```python
from build123d import *

# Parameters (mm, degrees)
F0_W      = 914.4
F0_H      = 812.8
F0_W_2    = 762
F0_H_2    = 609.6
F1_DEPTH  = 63.5
F2_W      = 914.4
F2_H      = 812.8
F2_W_2    = 762
F2_H_2    = 660.4
F3_DEPTH  = 1219.2
F5_DEPTH  = 812.8
F5_FACE_W = 762
F5_FACE_H = 76.2
F7_W      = 762
F7_H      = 282.4884019335
F9_DEPTH  = 76.2
F10_W     = 63.5
F10_H     = 76.2
F12_W     = 762
F12_H     = 279.4
F13_DEPTH = 88.9
F14_START = -330.2
F14_DEPTH = 152.4
F15_R     = 101.6
F16_DEPTH = 76.2
F17_DEPTH = 76.2


with BuildPart() as f1:
    # F0 (on Top) → F1 (new body)
    with BuildSketch(Plane.XY):
        Rectangle(F0_W, F0_H)
        Rectangle(F0_W_2, F0_H_2, mode=Mode.SUBTRACT)
        Rectangle(F0_W_2, F0_H_2)
    extrude(amount=F1_DEPTH)

    # F2 (on face) → F3 (join)
    with BuildSketch(Plane.XY.offset(63.5)):
        Rectangle(F2_W, F2_H)
        Rectangle(F2_W_2, F2_H_2, mode=Mode.SUBTRACT)
    extrude(amount=F3_DEPTH)

    # F4 (on face) → F5 (join, through all)
    with BuildSketch(Plane.XZ.offset(406.4)):
        with BuildLine():
            Line((381, 1282.7), (457.2, 1282.7))
            ThreePointArc((457.2, 1282.7), (364.8558540126, 1558.2214071405), (125.1263088683, 1722.4445245014))
            Line((125.1263088683, 1722.4445245014), (63.5, 1658.3710662268))
            ThreePointArc((63.5, 1658.3710662268), (290.9935566297, 1528.6344424842), (381, 1282.7))
        make_face()
        with BuildLine():
            ThreePointArc((-125.1263088683, 1722.4445245014), (-364.8558540126, 1558.2214071405), (-457.2, 1282.7))
            Line((-457.2, 1282.7), (-381, 1282.7))
            ThreePointArc((-381, 1282.7), (-290.9935566297, 1528.6344424842), (-63.5, 1658.3710662268))
            Line((-63.5, 1658.3710662268), (-125.1263088683, 1722.4445245014))
        make_face()
        with BuildLine():
            Line((63.5, 1658.3710662268), (125.1263088683, 1722.4445245014))
            ThreePointArc((125.1263088683, 1722.4445245014), (0, 1739.9), (-125.1263088683, 1722.4445245014))
            Line((-125.1263088683, 1722.4445245014), (-63.5, 1658.3710662268))
            ThreePointArc((-63.5, 1658.3710662268), (0, 1663.7), (63.5, 1658.3710662268))
        make_face()
    extrude(amount=-F5_DEPTH)

    # F5_face (on face) → F6 (join, up to the next surface of F1)
    with BuildSketch(Plane(origin=(0, 368.3, 1282.7), x_dir=(1, 0, 0), z_dir=(0, 0, 1))):
        Rectangle(F5_FACE_W, F5_FACE_H)
    extrude(until=Until.NEXT)

    # F5_face (on face) → F8 (join, up to the next surface of F1)
    with BuildSketch(Plane(origin=(0, 368.3, 1282.7), x_dir=(1, 0, 0), z_dir=(0, 0, 1))):
        with Locations((0, -736.6)):
            Rectangle(F5_FACE_W, F5_FACE_H)
    extrude(until=Until.NEXT)

    # F7 (on face) → F9 (cut, through all)
    with BuildSketch(Plane.XZ.offset(406.4)):
        with BuildLine():
            Line((381, 1282.7), (-381, 1282.7))
            Line((-381, 1282.7), (-381, 726.9884019335))
            ThreePointArc((-381, 726.9884019335), (0, 850.9), (381, 726.9884019335))
            Line((381, 726.9884019335), (381, 1282.7))
        make_face()
        with BuildLine():
            ThreePointArc((381, 650.7884019335), (0, 774.7), (-381, 650.7884019335))
            Line((-381, 650.7884019335), (381, 650.7884019335))
        make_face()
        with Locations((0, 509.5442009667)):
            Rectangle(F7_W, F7_H)
    extrude(amount=-F9_DEPTH, mode=Mode.SUBTRACT)

    # F11: sweep along a path in F7
    with BuildLine(Plane.XZ.offset(406.4)) as f11_path:
        ThreePointArc((381, 650.7884019335), (0, 774.7), (-381, 650.7884019335))
    # F10 (on face) → F11 (sweep)
    with BuildSketch(Plane.YZ.offset(-381)):
        with Locations((-152.4, 688.8884019335)):
            Rectangle(F10_W, F10_H)
        with Locations((88.9, 688.8884019335)):
            Rectangle(F10_W, F10_H)
        with Locations((298.45, 688.8884019335)):
            Rectangle(F10_W, F10_H)
    sweep(path=f11_path.line)

    # F12 (on face) → F13 (cut)
    with BuildSketch(Plane(origin=(0, 406.4, 0), x_dir=(-1, 0, 0), z_dir=(0, 1, 0))):
        with Locations((0, 203.2)):
            Rectangle(F12_W, F12_H)
    extrude(amount=-F13_DEPTH, mode=Mode.SUBTRACT)

    # F4 (on face) → F14 (cut)
    with BuildSketch(Plane.XZ.offset(406.4).offset(F14_START)):
        with BuildLine():
            Line((63.5, 1658.3710662268), (125.1263088683, 1722.4445245014))
            ThreePointArc((125.1263088683, 1722.4445245014), (0, 1739.9), (-125.1263088683, 1722.4445245014))
            Line((-125.1263088683, 1722.4445245014), (-63.5, 1658.3710662268))
            ThreePointArc((-63.5, 1658.3710662268), (0, 1663.7), (63.5, 1658.3710662268))
        make_face()
    extrude(amount=-F14_DEPTH, mode=Mode.SUBTRACT)

    # F15 (on face) → F16 (cut, through all)
    with BuildSketch(Plane(origin=(-457.2, 0, 0), x_dir=(0, -1, 0), z_dir=(-1, 0, 0))):
        with Locations((0, 509.5442009667)):
            Circle(F15_R)
    extrude(amount=-F16_DEPTH, mode=Mode.SUBTRACT)

    # F7 (on face) → F17 (join, through all)
    with BuildSketch(Plane.XZ.offset(406.4)):
        with BuildLine():
            ThreePointArc((381, 650.7884019335), (0, 774.7), (-381, 650.7884019335))
            Line((-381, 650.7884019335), (381, 650.7884019335))
        make_face()
    extrude(amount=-F17_DEPTH)


solid = f1.part
```
The model under review builds one solid part; all positions refer to its coordinate system, in mm. A direction names the side the tool comes from. Round coordinates to 2 decimals unless told otherwise and drop trailing zeros. Loops run counter-clockwise (first coordinate to the right, second up) from the corner with the lowest first, then second, coordinate; pieces in that order, holes last. Notation, with made-up numbers: (47.5, 89.25) -> (102.5, 89.25) arc R10 ccw to (102.5, 99.25) -> close; hole circle Ø2 at (88.25, 27). An arc over 180 degrees is marked (long way). Answer as a JSON object with one key per item and string values. Group by question number.
1) We need section C-C on x = 0. Give the number of separate pieces and of enclosed holes in the cut face, then the cut area to 3 significant figures.
2) For line 1 (X direction, y = 269, z = 316.5); line 2 (Y direction, x = -237, z = 359.5); line 3 (Z direction, x = 4, y = -109), list the stretches that pass through material, from the lowest coordinate up. Write a range as [from, to].
3) We need section B-B on y = 310. Write out the cut boundary in (x, z), then the cut area to 3 significant figures.
4) Mouldability with a two-part tool opening along X and no side actions: class faces 6 (the face through (5, -369, 1282.7)), 7 (the face through (-6, 6, 0)), 8 (the face through (457.2, -6, 632)) as released by +X, released by -X, zero draft, split by the parting line, or undercut.
5) For faces 1 (the face through (5.702, 298.894, 774.675)), 2 (the face through (-5, -369, 368.3)), 3 (the face through (-94.745, -1.067, 1690.856)), 4 (the face through (-419.633, -54.62, 595.214)), 5 (the face through (-5, 43, 63.5)), list the 3-axis set-ups (+Z, -Z, +X, -X, +Y, -Y) from which the entire face can be reached by the end or side of a thin tool; tool diameter is ignored.
6) For pin 1 Ø2 at (x, z) = (-141.5, 619.5) entering from -Y, flat-tipped, find the tip position at first contact; note if it passes through.
7) We need section A-A on y = 0. Write out the cut boundary in (x, z).
Result set:
{
 "1": {"separate pieces": "6", "enclosed holes": "0", "area": "282,000 mm²"},
 "2": {"line 1": "[-457.2, -381], [381, 457.2]", "line 2": "[-406.4, -330.2], [330.2, 406.4]", "line 3": "[0, 63.5], [1663.68, 1739.88]"},
 "3": {"outline": "(-457.2, 0) -> (457.2, 0) -> (457.2, 1282.7) arc R457.2 ccw to (-457.2, 1282.7) -> close; hole (-381, 63.5) -> (381, 63.5) -> (381, 650.79) arc R647.7 ccw to (-381, 650.79) -> close; hole (-381, 726.99) arc R710.74 cw to (381, 726.99) -> (381, 1282.7) arc R381 ccw to (-381, 1282.7) -> close", "area": "395,000 mm²"},
 "4": {"face 6": "undercut", "face 7": "zero draft", "face 8": "released by +X"},
 "5": {"face 1": "none", "face 2": "-Y", "face 3": "+Z", "face 4": "-X", "face 5": "+Y"},
 "6": {"pin 1": "y = 330.2"},
 "7": {"outline": "(-457.2, 0) -> (457.2, 0) -> (457.2, 1282.7) arc R457.2 ccw to (125.13, 1722.44) -> (63.5, 1658.37) arc R381 cw to (381, 1282.7) -> (381, 63.5) -> (-381, 63.5) -> (-381, 407.94) -> (-457.2, 407.94) -> close; (-457.2, 611.14) -> (-381, 611.14) -> (-381, 1282.7) arc R381 cw to (-63.5, 1658.37) -> (-125.13, 1722.44) arc R457.2 ccw to (-457.2, 1282.7) -> close"}
}
